Work out the finished part from the listing and answer in its coordinate system (mm). Face numbers are marked on the shaded views. A direction names the side the tool comes from. Round coordinates to 2 decimals unless told otherwise and drop trailing zeros. Loops run counter-clockwise (first coordinate to the right, second up) from the corner with the lowest first, then second, coordinate; pieces in that order, holes last.
from build123d import *

# Parameters (mm, degrees)
CUT_EXTRUDE1_DEPTH             = 59.345951016
CUT_EXTRUDE3_DEPTH             = 5.5
SKETCH10_W                     = 20
SKETCH10_H                     = 5.5
CUT_EXTRUDE5_DEPTH             = 10
F_1_5_1_5_DIAMETER_HOLE1_D     = 1.5
F_1_5_1_5_DIAMETER_HOLE1_DEPTH = 3.227722445
SKETCH12_W                     = 3.119585898
SKETCH12_H                     = 5.5
CUT_EXTRUDE6_DEPTH             = 66.759029798
FILLET1_R                      = 1


with BuildPart() as part:
    # Sketch2 → Revolve1 (revolve)
    with BuildSketch(Plane(origin=(0, 0, 0), x_dir=(0, 0, -1), z_dir=(1, 0, 0))):
        Polygon((0, 0), (41, 0), (41, -1), (38, -1), (38, -6.5), (0, -6.5), align=None)
    revolve(axis=Axis((0, -6.5, 0), (0, 1, 0)))

    # Sketch3 → Cut-Extrude1 (cut, through all)
    with BuildSketch(Plane(origin=(0, 0, 0), x_dir=(1, 0, 0), z_dir=(0, 1, 0))):
        with BuildLine():
            Line((-13.453624047, -32.310988843), (13.453624047, -32.310988843))
            ThreePointArc((13.453624047, -32.310988843), (23.418599656, 26.010943661), (-33.541019662, 10))
            Line((-33.541019662, 10), (-33.541019662, -10))
            ThreePointArc((-33.541019662, -10), (-26.010943661, -23.418599656), (-13.453624047, -32.310988843))
        make_face()
    extrude(amount=-CUT_EXTRUDE1_DEPTH, mode=Mode.SUBTRACT)

    # Sketch6 → Cut-Extrude3 (cut)
    with BuildSketch(Plane.XZ.offset(6.5)):
        with BuildLine():
            Line((-13.453624047, 35.538711288), (13.453624047, 35.538711288))
            ThreePointArc((13.453624047, 35.538711288), (0, 38), (-13.453624047, 35.538711288))
        make_face()
        with BuildLine():
            Line((-36.66060556, -10), (-36.66060556, 10))
            ThreePointArc((-36.66060556, 10), (-38, 0), (-36.66060556, -10))
        make_face()
    extrude(amount=-CUT_EXTRUDE3_DEPTH, mode=Mode.SUBTRACT)

    # Sketch10 → Cut-Extrude5 (cut)
    with BuildSketch(Plane.ZY.offset(36.66060556)):
        with Locations((0, -3.75)):
            Rectangle(SKETCH10_W, SKETCH10_H)
    extrude(amount=-CUT_EXTRUDE5_DEPTH, mode=Mode.SUBTRACT)

    # Ø1.5 (1.5) Diameter Hole1
    with Locations(Plane.XY.offset(35.538711288)):
        with Locations((9.453624047, -3.75), (5.453624047, -3.75), (-5.453624047, -3.75), (-9.453624047, -3.75)):
            Hole(F_1_5_1_5_DIAMETER_HOLE1_D / 2, depth=F_1_5_1_5_DIAMETER_HOLE1_DEPTH)

    # Sketch12 → Cut-Extrude6 (cut, through all)
    with BuildSketch(Plane.XY.offset(-10)):
        with Locations((-35.100812611, -3.75)):
            Rectangle(SKETCH12_W, SKETCH12_H)
    extrude(amount=-CUT_EXTRUDE6_DEPTH, mode=Mode.SUBTRACT)

    # Fillet1
    fillet1_edges = [part.edges().sort_by_distance(p)[0] for p in [
        (-28.123218981, -1, 25.555519055),
        (0, -1, 35.538711288),
        (28.526245907, -1, -25.104846036),
    ]]
    fillet(fillet1_edges, radius=FILLET1_R)


solid = part.part
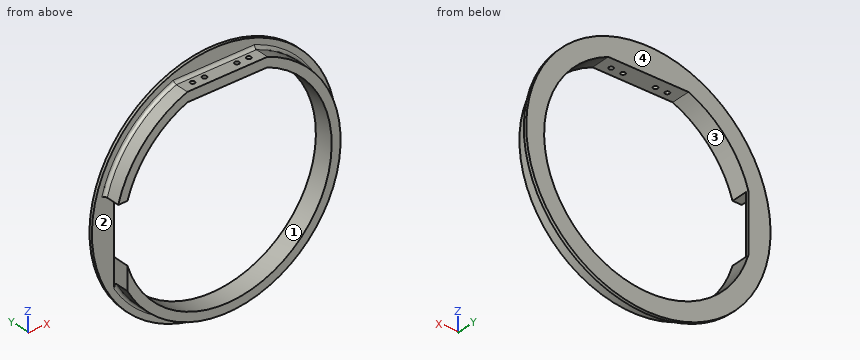
Item 1: Each of these flat-tipped pins is pushed along its axis until it touches: P1, Ø2, axis at x = -5.45, y = -3.75, coming from the +Z side; P2, Ø2, axis at x = 5.5, z = -32, coming from the -Y side; P3, Ø2, axis at x = -36.5, y = -3.5, coming from the -Z side; P4, Ø1.2, axis at x = 9.45, y = -3.75, coming from the -Z side. Where does it stop, or does it pass through?
Item 2: Determine the mould class of the marked faces 3 and 4 for opening direction Z: pulls with the +Z half, pulls with the -Z half, needs draft (parallel to the pull), parting line crosses it, or undercut.
Item 3: Straight lines are drawn through the part: line 1 (Z direction, x = 0, y = -2); line 2 (Z direction, x = -1, y = -0.25); line 3 (X direction, y = -3.5, z = 31.5). For each, find the intervals that lie inside material, in ascending order.
Item 4: Section A-A, the plane x = 0 is taken. Give the vertices of the cut face in (y, z), plus the area to 3 significant figures.
Item 5: For the marked faces 1 and 2, determine the directions among +Z, -Z, +X, -X, +Y, -Y from which every point of the face is accessible in a straight line to the end or side of a thin tool.
Item 6: Section B-B, the plane z = 0 is taken. Give the vertices of the cut face in (x, y).
Answer below:
1. P1: stops at z = 35.54
1. P2: passes through
1. P3: stops at z = 10
1. P4: stops at z = -36.96
2. face 3: undercut
2. face 4: needs draft
3. line 1: z = -38 to -35, 32.31 to 35.54
3. line 2: z = -40.99 to -34.99, 32.31 to 40.99
3. line 3: x = -21.25 to -15.26, 15.26 to 21.25
4. outline: (-6.5, -38) - (-2, -38) arc R1 cw to (-1, -39) - (-1, -41) - (0, -41) - (0, -35) - (-6.5, -35) - close; (-6.5, 32.31) - (0, 32.31) - (0, 41) - (-1, 41) - (-1, 36.54) arc R1 cw to (-2, 35.54) - (-6.5, 35.54) - close
4. area: 49.4 mm2
5. face 1: +Y, -Y
5. face 2: -Y
6. outline: (-41, -1) - (-33.54, -1) - (-33.54, 0) - (-41, 0) - close; (35, -6.5) - (38, -6.5) - (38, -2) arc R1 cw to (39, -1) - (41, -1) - (41, 0) - (35, 0) - close
